```python
from build123d import *

# Parameters (mm, degrees)
SALIENTE_EXTRUIR1_DEPTH = 5
CROQUIS2_R              = 16
CORTAR_EXTRUIR1_DEPTH   = 10
CROQUIS4_R              = 2.6
CORTAR_EXTRUIR2_DEPTH   = 10
MATRIZC1_COUNT          = 6
REDONDEO1_R             = 10
CROQUIS5_R              = 16
CORTAR_EXTRUIR3_DEPTH   = 282.780056072
CORTAR_EXTRUIR4_DEPTH   = 282.780056072
REDONDEO2_R             = 5
CROQUIS7_R              = 2.5
CORTAR_EXTRUIR5_DEPTH   = 10
CROQUIS8_R              = 2.5
CORTAR_EXTRUIR6_DEPTH   = 282.780056072
SKETCH1_R               = 4
CUT_EXTRUDE1_DEPTH      = 10
SKETCH2_R               = 2.5
CUT_EXTRUDE2_DEPTH      = 282.780056072
CIRPATTERN1_COUNT       = 4
SKETCH3_R               = 16
SKETCH3_R_2             = 6.5
BOSS_EXTRUDE1_DEPTH     = 10


with BuildPart() as part:
    # Croquis1 → Saliente-Extruir1 (new, symmetric)
    with BuildSketch(Plane(origin=(0, 0, 0), x_dir=(1, 0, 0), z_dir=(0, 1, 0))):
        with BuildLine():
            Line((-250, 30), (250, 30))
            Line((250, 30), (280, 30))
            Line((280, 30), (280, 0))
            Line((280, 0), (280, -30))
            Line((280, -30), (250, -30))
            Line((250, -30), (-250, -30))
            ThreePointArc((-250, -30), (-280, 0), (-250, 30))
        make_face()
    extrude(amount=SALIENTE_EXTRUIR1_DEPTH, both=True)

    # Croquis2 → Cortar-Extruir1 (cut)
    with BuildSketch(Plane(origin=(0, 5, 0), x_dir=(1, 0, 0), z_dir=(0, 1, 0))):
        with Locations(Location((-250, 0, 0), (0, 0, 270))):
            Circle(CROQUIS2_R)
    extrude(amount=-CORTAR_EXTRUIR1_DEPTH, mode=Mode.SUBTRACT)

    # Croquis4 → Cortar-Extruir2 (cut)
    with BuildSketch(Plane(origin=(0, 5, 0), x_dir=(1, 0, 0), z_dir=(0, 1, 0))):
        with Locations(Location((-250, 25, 0), (0, 0, 270))):
            Circle(CROQUIS4_R)
    cortar_extruir2 = extrude(amount=-CORTAR_EXTRUIR2_DEPTH, mode=Mode.SUBTRACT)

    # MatrizC1: Cortar-Extruir2 ×6 about axis
    matrizc1_axis = Axis((-250, 0, 0), (0, 1, 0))
    for i in range(1, MATRIZC1_COUNT):
        add(cortar_extruir2.rotate(matrizc1_axis, i * 360 / MATRIZC1_COUNT), mode=Mode.SUBTRACT)

    # Redondeo1
    redondeo1_edges = [part.edges().sort_by_distance(p)[0] for p in [
        (280, 0, -30),
        (280, 0, 30),
    ]]
    fillet(redondeo1_edges, radius=REDONDEO1_R)

    # Croquis5 → Cortar-Extruir3 (cut, through all)
    with BuildSketch(Plane(origin=(0, 5, 0), x_dir=(1, 0, 0), z_dir=(0, 1, 0))):
        with Locations(Location((230, 0, 0), (0, 0, 270))):
            Circle(CROQUIS5_R)
    extrude(amount=-CORTAR_EXTRUIR3_DEPTH, mode=Mode.SUBTRACT)

    # Croquis6 → Cortar-Extruir4 (cut, through all)
    with BuildSketch(Plane(origin=(0, 5, 0), x_dir=(1, 0, 0), z_dir=(0, 1, 0))):
        with BuildLine():
            Line((260, 30), (260, -30))
            Line((260, -30), (270, -30))
            ThreePointArc((270, -30), (277.071067812, -27.071067812), (280, -20))
            Line((280, -20), (280, 20))
            ThreePointArc((280, 20), (277.071067812, 27.071067812), (270, 30))
            Line((270, 30), (260, 30))
        make_face()
    extrude(amount=-CORTAR_EXTRUIR4_DEPTH, mode=Mode.SUBTRACT)

    # Redondeo2
    redondeo2_edges = [part.edges().sort_by_distance(p)[0] for p in [
        (260, 0, 30),
        (260, 0, -30),
    ]]
    fillet(redondeo2_edges, radius=REDONDEO2_R)

    # Croquis7 → Cortar-Extruir5 (cut)
    with BuildSketch(Plane.XZ.offset(5)):
        with Locations(Location((182.85, -22.5, 0), (0, 0, 270))):
            Circle(CROQUIS7_R)
        with Locations(Location((182.85, 22.5, 0), (0, 0, 270))):
            Circle(CROQUIS7_R)
    extrude(amount=-CORTAR_EXTRUIR5_DEPTH, mode=Mode.SUBTRACT)

    # Croquis8 → Cortar-Extruir6 (cut, through all)
    with BuildSketch(Plane.XZ.offset(5)):
        with Locations(Location((-202.85, -22.5, 0), (0, 0, 270))):
            Circle(CROQUIS8_R)
        with Locations(Location((-202.85, 22.5, 0), (0, 0, 270))):
            Circle(CROQUIS8_R)
    extrude(amount=-CORTAR_EXTRUIR6_DEPTH, mode=Mode.SUBTRACT)

    # Sketch1 → Cut-Extrude1 (cut)
    with BuildSketch(Plane(origin=(0, -5, 0), x_dir=(-1, 0, 0), z_dir=(0, -1, 0))):
        with Locations(Location((10, -22.5, 0), (0, 0, 90))):
            Circle(SKETCH1_R)
    cut_extrude1 = extrude(amount=-CUT_EXTRUDE1_DEPTH, mode=Mode.SUBTRACT)

    # Mirror1: Cut-Extrude1 across plane
    add(cut_extrude1.mirror(Plane.XY), mode=Mode.SUBTRACT)

    # Sketch2 → Cut-Extrude2 (cut, through all)
    with BuildSketch(Plane(origin=(0, 5, 0), x_dir=(1, 0, 0), z_dir=(0, 1, 0))):
        with Locations(Location((230, 24, 0), (0, 0, 270))):
            Circle(SKETCH2_R)
    cut_extrude2 = extrude(amount=-CUT_EXTRUDE2_DEPTH, mode=Mode.SUBTRACT)

    # CirPattern1: Cut-Extrude2 ×4 about axis
    cirpattern1_axis = Axis((230, 0, 0), (0, 1, 0))
    for i in range(1, CIRPATTERN1_COUNT):
        add(cut_extrude2.rotate(cirpattern1_axis, i * 360 / CIRPATTERN1_COUNT), mode=Mode.SUBTRACT)

    # Sketch3 → Boss-Extrude1 (add)
    with BuildSketch(Plane(origin=(0, 5, 0), x_dir=(1, 0, 0), z_dir=(0, 1, 0))):
        with Locations((230, 0)):
            Circle(SKETCH3_R)
        with Locations(Location((230, 0, 0), (0, 0, 270))):
            Circle(SKETCH3_R_2, mode=Mode.SUBTRACT)
    extrude(amount=-BOSS_EXTRUDE1_DEPTH)


solid = part.part
```
Design review of the part built by this model. Coordinates are the model's own, in mm. Coordinates: 2 decimals unless noted, no trailing zeros.
Q1. We need section A-A on y = -1.25. State how many separate pieces and enclosed holes the cut face has, and give its area (3 significant figures).
Reported:
separate pieces: 1
enclosed holes: 18
area: 30,700 mm2
Q2. The part is to be moulded in two halves that separate along Z. For faces 1 (the face through (223.655, 0.07, -1.409)), 2 (the face through (6, 0, 30)), 3 (the face through (260, 0, 0)), say which applies: +Z half, -Z half, draft (parallel to the pull), parting line (faces both ways), or undercut.
Reported:
face 1: undercut
face 2: +Z half
face 3: draft
Q3. For pin 1 (6 mm diameter, centred on x = -228.35, z = -12.5, fed in from -Y); pin 2 (3 mm diameter, centred on x = 230, z = 24, fed in from +Y), all flat-tipped, find the tip position at first contact; note any pin that passes through.
Reported:
pin 1: stops at y = -5
pin 2: passes through
Q4. To check wall thickness, follow line 1 (X direction, y = -4.25, z = -12); line 2 (Z direction, x = -202.85, y = -2.5); line 3 (X direction, y = 1.5, z = 12.5). State the ranges of each line that lie inside material, in increasing order.
Reported:
line 1: x = -277.5 to -274.2, -269.1 to -260.58, -239.42 to -230.9, -225.8 to 260
line 2: z = -30 to -25, -20 to 20, 25 to 30
line 3: x = -277.27 to -274.25, -269.05 to -259.99, -240.01 to -230.95, -225.75 to 260
